from build123d import *

# Parameters (mm, degrees)
SKETCH_W      = 191.3
SKETCH_H      = 69.5
PAD_DEPTH     = 1.6
SKETCH002_R   = 1.75
SKETCH002_R_2 = 6.1
SKETCH002_W   = 107
SKETCH002_H   = 50
SKETCH002_W_2 = 18
SKETCH002_H_2 = 32
POCKET_DEPTH  = 1.601


with BuildPart() as part:
    # Sketch → Pad (new body)
    with BuildSketch(Plane.XY):
        with Locations((95.65, 34.75)):
            Rectangle(SKETCH_W, SKETCH_H)
    extrude(amount=PAD_DEPTH)

    # Sketch002 (on Face6 of Pad) → Pocket (cut, through all)
    with BuildSketch(Plane.XY.offset(1.6)):
        with Locations((184.15, 4.5)):
            Circle(SKETCH002_R)
        with Locations((52.15, 4.5)):
            Circle(SKETCH002_R)
        with Locations((184.15, 64.5)):
            Circle(SKETCH002_R)
        with Locations((52.15, 64.5)):
            Circle(SKETCH002_R)
        with Locations((19.15, 11.5)):
            Circle(SKETCH002_R)
        with Locations((19.15, 39.5)):
            Circle(SKETCH002_R)
        with Locations((45.15, 11.5)):
            Circle(SKETCH002_R)
        with Locations((45.15, 39.5)):
            Circle(SKETCH002_R)
        with Locations((20.9, 55.5)):
            Circle(SKETCH002_R_2)
        with Locations((119.65, 36)):
            Rectangle(SKETCH002_W, SKETCH002_H)
        with Locations((32.15, 25.5)):
            Rectangle(SKETCH002_W_2, SKETCH002_H_2)
    extrude(amount=-POCKET_DEPTH, mode=Mode.SUBTRACT)


solid = part.part
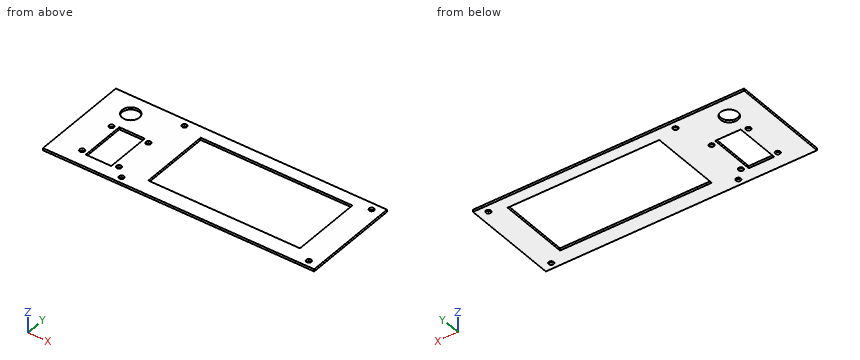
Here's how the part is built. I have some questions about the finished solid (model axes, mm). Coordinates: 2 decimals unless noted, no trailing zeros. Write each loop counter-clockwise with the first axis right and the second up, starting at its lowest first coordinate (ties: lowest second). Pieces come first, ordered by that corner, then holes.
1) If we section it at A-A (x = 52.15): List the corners of the cut face in (y, z) for me.
Filled in:
outline: (0, 0) - (2.75, 0) - (2.75, 1.6) - (0, 1.6) - close; (6.25, 0) - (62.75, 0) - (62.75, 1.6) - (6.25, 1.6) - close; (66.25, 0) - (69.5, 0) - (69.5, 1.6) - (66.25, 1.6) - close
2) If I drill on line 1 (X direction, y = 18, z = 0.5); line 2 (Y direction, x = 52.15, z = 0.45); line 3 (X direction, y = 64.5, z = 0.5), over which ranges is the centre line in solid material (lowest first)?
Filled in:
line 1: x = 0 to 23.15, 41.15 to 66.15, 173.15 to 191.3
line 2: y = 0 to 2.75, 6.25 to 62.75, 66.25 to 69.5
line 3: x = 0 to 50.4, 53.9 to 182.4, 185.9 to 191.3
3) If we section it at B-B (y = 34): List the corners of the cut face in (x, z) for me.
Filled in:
outline: (0, 0) - (23.15, 0) - (23.15, 1.6) - (0, 1.6) - close; (41.15, 0) - (66.15, 0) - (66.15, 1.6) - (41.15, 1.6) - close; (173.15, 0) - (191.3, 0) - (191.3, 1.6) - (173.15, 1.6) - close
4) If we section it at C-C (z = 0.35): Count the separate pieces of the cut face and the enclosed holes in it, plus the area to 3 significant figures.
Filled in:
separate pieces: 1
enclosed holes: 11
area: 7,180 mm2
5) I'm going to push flat-ended pins straight in: pin 1 (10 mm diameter, centred on x = 165.5, y = 20.5, fed in from +Z); pin 2 (4 mm diameter, centred on x = 45.15, y = 39.5, fed in from +Z). Where does each tip first touch, or does it pass through?
Filled in:
pin 1: passes through
pin 2: stops at z = 1.6
6) If we section it at D-D (x = 71.5): List the corners of the cut face in (y, z) for me, plus the area to 3 significant figures.
Filled in:
outline: (0, 0) - (11, 0) - (11, 1.6) - (0, 1.6) - close; (61, 0) - (69.5, 0) - (69.5, 1.6) - (61, 1.6) - close
area: 31.2 mm2
